Verification items for the finished model (mm, model axes). A direction names the side the tool comes from. Coordinates: 2 decimals unless noted, no trailing zeros. Loops run counter-clockwise (first coordinate to the right, second up) from the corner with the lowest first, then second, coordinate; pieces in that order, holes last.
Q1. Sectioned sample at B-B (x = -4). Enter the section's corners in (y, z), then the cut area to 3 significant figures.
Q2. Sectioned sample at A-A (z = 3.5). Enter the section's corners in (x, y), then the cut area to 3 significant figures.
Q3. Access from +Z, -Z, +X, -X, +Y, -Y to the whole of each face (thin tool, end or side, straight path). Record for faces 4 (the face through (0, 16.891, 17)), 5 (the face through (-17, 0, 2.54)).
Q4. Mould release check, pull along Y, two halves, no side actions. Record for faces 1 (the face through (0, -14.351, 19)), 2 (the face through (0, -16.891, 17)), 3 (the face through (-2, -15, 35.306)): +Y half, -Y half, draft (parallel to the pull), parting line (faces both ways), or undercut.
Q5. Sectioned sample at D-D (x = 21.5). Enter the section's corners in (y, z), then the cut area to 3 significant figures.
Q6. Go/stop test with a flat-tipped pin: P1, Ø11.5, axis at x = -12.5, y = -1, coming from the +Z side. Record where the tip stops, or that it passes through.
Q7. Material ranges on probe 1 along X at (y, z) = (-2, 5); probe 2 along Y at (x, z) = (0, 0.75), recorded low to high.
Q8. Sectioned sample at C-C (y = 0). Enter the section's corners in (x, z).
```python
from build123d import *

# Parameters (mm, degrees)
F0_W     = 50.8
F0_H     = 33.782
F1_DEPTH = 35.306
F2_T     = -2.54
F3_R     = 14.351
F4_DEPTH = 25.4


with BuildPart() as f1:
    # F0 (on Top) → F1 (new body)
    with BuildSketch(Plane.XY):
        Rectangle(F0_W, F0_H)
    extrude(amount=F1_DEPTH)

    # F2
    f2_openings = [f1.faces().sort_by_distance(p)[0] for p in [
        (0, 0, 35.306),
    ]]
    offset(amount=F2_T, openings=f2_openings)

    # F3 (on face) → F4 (cut)
    with BuildSketch(Plane(origin=(0, 0, 0), x_dir=(1, 0, 0), z_dir=(0, 0, -1))):
        Circle(F3_R)
    extrude(amount=-F4_DEPTH, mode=Mode.SUBTRACT)


solid = f1.part
```
Geometry check:
1. outline: (-16.89, 0) - (-13.78, 0) - (-13.78, 2.54) - (-14.35, 2.54) - (-14.35, 35.31) - (-16.89, 35.31) - close; (13.78, 0) - (16.89, 0) - (16.89, 35.31) - (14.35, 35.31) - (14.35, 2.54) - (13.78, 2.54) - close
1. area: 182 mm2
2. outline: (-25.4, -16.89) - (25.4, -16.89) - (25.4, 16.89) - (-25.4, 16.89) - close; hole (-22.86, -14.35) - (22.86, -14.35) - (22.86, 14.35) - (-22.86, 14.35) - close
2. area: 404 mm2
3. face 4: +Z, -Z, +X, -X, +Y
3. face 5: +Z
4. face 1: undercut
4. face 2: -Y half
4. face 3: draft
5. outline: (-16.89, 0) - (16.89, 0) - (16.89, 35.31) - (14.35, 35.31) - (14.35, 2.54) - (-14.35, 2.54) - (-14.35, 35.31) - (-16.89, 35.31) - close
5. area: 252 mm2
6. P1: stops at z = 2.54
7. probe 1: x = -25.4 to -22.86, 22.86 to 25.4
7. probe 2: y = -16.89 to -14.35, 14.35 to 16.89
8. outline: (-25.4, 0) - (-14.35, 0) - (-14.35, 2.54) - (-22.86, 2.54) - (-22.86, 35.31) - (-25.4, 35.31) - close; (14.35, 0) - (25.4, 0) - (25.4, 35.31) - (22.86, 35.31) - (22.86, 2.54) - (14.35, 2.54) - close
